Read the model definition and answer for the solid it produces. Units are mm, in the model's axes. Face numbers are marked on the shaded views. A direction names the side the tool comes from. Give positions to 0.01 mm unless a question says otherwise; leave off trailing zeros. Order: outer loops, then holes, each group sorted by start corner. A loop starts at its lowest first (then second) coordinate and runs counter-clockwise, first axis right, second up. Notation, with made-up numbers: (27, -31.5) - (82, -31.5) arc R12 ccw to (82, -13.5) - close; hole circle Ø9 at (4, 31.25). An arc over 180 degrees is marked (long way). Return JSON: item names as keys, results as strings.
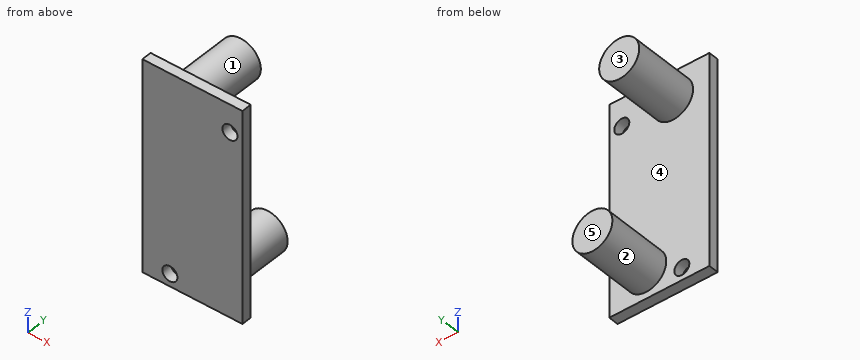
```python
from build123d import *

# Parameters (mm, degrees)
SKETCH1_W           = 20
SKETCH1_H           = 42
BOSS_EXTRUDE1_DEPTH = 2
SKETCH2_R           = 4
BOSS_EXTRUDE2_DEPTH = 13
SKETCH3_R           = 1.5
CUT_EXTRUDE1_DEPTH  = 27.645825189


with BuildPart() as part:
    # Sketch1 → Boss-Extrude1 (new body)
    with BuildSketch(Plane(origin=(0, 0, 0), x_dir=(1, 0, 0), z_dir=(0, 1, 0))):
        Rectangle(SKETCH1_W, SKETCH1_H)
    extrude(amount=BOSS_EXTRUDE1_DEPTH)

    # Sketch2 → Boss-Extrude2 (add)
    with BuildSketch(Plane(origin=(0, 2, 0), x_dir=(1, 0, 0), z_dir=(0, 1, 0))):
        with Locations(Location((2.611238323, 15.696088344, 0), (0, 0, 90))):
            Circle(SKETCH2_R)
        with Locations(Location((-2.7484016, -15.525941045, 0), (0, 0, 90))):
            Circle(SKETCH2_R)
    extrude(amount=BOSS_EXTRUDE2_DEPTH)

    # Sketch3 → Cut-Extrude1 (cut, through all)
    with BuildSketch(Plane(origin=(0, 2, 0), x_dir=(1, 0, 0), z_dir=(0, 1, 0))):
        with Locations(Location((-4.5, 18.5, 0), (0, 0, 270))):
            Circle(SKETCH3_R)
        with Locations(Location((7.5, -15.5, 0), (0, 0, 270))):
            Circle(SKETCH3_R)
    extrude(amount=-CUT_EXTRUDE1_DEPTH, mode=Mode.SUBTRACT)


solid = part.part
```
Q1. Given pin 1 (2.5 mm diameter, centred on x = -4.5, z = -18.5, fed in from -Y); pin 2 (1.5 mm diameter, centred on x = 0.5, y = 3, fed in from +Z); pin 3 (5 mm diameter, centred on y = 11, z = 16, fed in from -X), each flat-ended and moving along its own axis, determine where each tip first touches the part or whether it passes through.
Values:
{"pin 1": "passes through", "pin 2": "stops at z = 18.65", "pin 3": "stops at x = -6.75"}
Q2. A cutting plane is placed at B-B (z = -18.5). Write down the section's boundary in (x, y).
Values:
{"outline": "(-10, 0) - (-6, 0) - (-6, 2) - (-10, 2) - close; (-3, 0) - (10, 0) - (10, 2) - (5.46, 2) - (5.46, 15) - (-0.24, 15) - (-0.24, 2) - (-3, 2) - close"}
Q3. Consider L1, parallel to X at y = 1, z = 15.5; L2, parallel to X at y = 0.4, z = -18.5; L3, parallel to Y at x = 2.75, z = 3.5. Determine where each line is inside the solid, lowest interval first.
Values:
{"L1": "x = -10 to 6, 9 to 10", "L2": "x = -10 to -6, -3 to 10", "L3": "y = 0 to 2"}
Q4. A cutting plane is placed at C-C (x = 0.25). Write down the section's boundary in (y, z).
Values:
{"outline": "(0, -21) - (2, -21) - (2, -18.92) - (15, -18.92) - (15, -12.47) - (2, -12.47) - (2, 12.88) - (15, 12.88) - (15, 18.17) - (2, 18.17) - (2, 21) - (0, 21) - close"}
Q5. A cutting plane is placed at D-D (y = 10). Write down the section's boundary in (x, z), and give its area (3 significant figures).
Values:
{"outline": "circle Ø8 at (-2.75, 15.53); circle Ø8 at (2.61, -15.7)", "area": "101 mm²"}
Q6. Determine the mould class of the marked faces 1, 2 and 3 for opening direction Z: released by +Z, released by -Z, zero draft, split by the parting line, or undercut.
Values:
{"face 1": "undercut", "face 2": "undercut", "face 3": "zero draft"}
Q7. For the marked faces 4 and 5, determine the directions among +Z, -Z, +X, -X, +Y, -Y from which every point of the face is accessible in a straight line to the end or side of a thin tool.
Values:
{"face 4": "+Y", "face 5": "+Z, -Z, +X, -X, +Y"}
Q8. A cutting plane is placed at A-A (x = 7.5). Write down the section's boundary in (y, z).
Values:
{"outline": "(0, -21) - (2, -21) - (2, 14) - (0, 14) - close; (0, 17) - (2, 17) - (2, 21) - (0, 21) - close"}
